```python
from build123d import *

# Parameters (mm, degrees)
F0_W     = 82.55
F0_H     = 57.15
F0_W_2   = 76.2
F0_H_2   = 50.8
F1_DEPTH = 152.4
F2_W     = 6.35
F2_H     = 57.15
F3_DEPTH = 50.8
F4_W     = 50.8
F4_H     = 6.35
F5_DEPTH = 50.8
F7_DEPTH = 118.618


with BuildPart() as f1:
    # F0 (on Front) → F1 (new body)
    with BuildSketch(Plane.XZ):
        with Locations((3.728271, -19.37303)):
            Rectangle(F0_W, F0_H)
        with Locations((3.728271, -19.37303)):
            Rectangle(F0_W_2, F0_H_2, mode=Mode.SUBTRACT)
    extrude(amount=F1_DEPTH)

    # F2 (on face) → F3 (join)
    with BuildSketch(Plane.YZ.offset(45.003271)):
        with Locations((-3.175, -19.37303)):
            Rectangle(F2_W, F2_H)
    extrude(amount=F3_DEPTH)

    # F4 (on face) → F5 (join)
    with BuildSketch(Plane.XZ.offset(6.35)):
        with Locations((70.403271, -44.77303)):
            Rectangle(F4_W, F4_H)
        with Locations((70.403271, 6.02697)):
            Rectangle(F4_W, F4_H)
    extrude(amount=F5_DEPTH)

    # F6 (on face) → F7 (cut)
    with BuildSketch(Plane.XY.offset(9.20197)):
        Polygon((95.803271, -6.35), (45.003271, -57.15), (95.803271, -57.15), align=None)
    extrude(amount=-F7_DEPTH, mode=Mode.SUBTRACT)


solid = f1.part
```
Input: part model. Units: mm. Frame: model coordinates. A direction names the side the tool comes from. Give positions to 0.01 mm unless a question says otherwise; leave off trailing zeros. Order: outer loops, then holes, each group sorted by start corner. A loop starts at its lowest first (then second) coordinate and runs counter-clockwise, first axis right, second up. Notation, with made-up numbers: M 61.5,67.25 L 112.5,67.25 A19 cw 112.5,71.25 Z; hole C 82.25,26.25 d4. An arc over 180 degrees is marked long. Return JSON: item names as keys, results as strings.
Item 1: Ray query, probe 1 along X at (y, z) = (-30.5, -10.5); probe 2 along Z at (x, y) = (-23.5, -36); probe 3 along X at (y, z) = (-21.5, 4.5). Return the intervals inside material, ascending.
Solutions:
{"probe 1": "-37.55 to -34.37, 41.83 to 45", "probe 2": "-47.95 to -44.77, 6.03 to 9.2", "probe 3": "-37.55 to -34.37, 41.83 to 80.65"}
Item 2: Cut plane D-D (x = 62). Return loops of the section in (y, z), then the cut area to 3 significant figures.
Solutions:
{"outline": "M -40.15,-47.95 L 0,-47.95 L 0,9.2 L -40.15,9.2 L -40.15,2.85 L -6.35,2.85 L -6.35,-41.6 L -40.15,-41.6 Z", "area": "792 mm^2"}
Item 3: Pull-direction query (X, two-part tool) for faces 1 (the flat face through (95.803, -3, -20)), 2 (the flat face through (-37.547, -75, -20)), 3 (the flat face through (3, -75, -44.773)), 4 (the flat face through (41.828, -75, -20)); classes: +X half, -X half, draft (parallel to the pull), parting line (faces both ways), or undercut.
Solutions:
{"face 1": "+X half", "face 2": "-X half", "face 3": "undercut", "face 4": "undercut"}
Item 4: Cut plane B-B (x = -1.5). Return loops of the section in (y, z).
Solutions:
{"outline": "M -152.4,-47.95 L 0,-47.95 L 0,-44.77 L -152.4,-44.77 Z; M -152.4,6.03 L 0,6.03 L 0,9.2 L -152.4,9.2 Z"}
Item 5: Cut plane C-C (y = -83). Return loops of the section in (x, z).
Solutions:
{"outline": "M -37.55,-47.95 L 45,-47.95 L 45,9.2 L -37.55,9.2 Z; hole M -34.37,-44.77 L 41.83,-44.77 L 41.83,6.03 L -34.37,6.03 Z"}
Item 6: Cut plane A-A (z = -11.5). Return loops of the section in (x, y).
Solutions:
{"outline": "M -37.55,-152.4 L -34.37,-152.4 L -34.37,0 L -37.55,0 Z; M 41.83,-152.4 L 45,-152.4 L 45,-6.35 L 95.8,-6.35 L 95.8,0 L 41.83,0 Z"}
Item 7: Access query for faces 5 (the flat face through (3, -75, 6.027)), 6 (the flat face through (13, -75, -47.948)), 7 (the flat face through (45.003, -78, -20)). Directions: +Z, -Z, +X, -X, +Y, -Y. A direction counts if a zero-diameter tool reaches every point of the face in a straight line with its end or side. Return the directions, or none.
Solutions:
{"face 5": "+Y, -Y", "face 6": "-Z, +X, -X, +Y, -Y", "face 7": "+X, -Y"}
Item 8: First-contact query: P1, Ø4, axis at x = 79.5, z = 0, coming from the -Y side; P2, Ø5, axis at y = -110.5, z = -8.5, coming from the +X side. Flat tips, straight axial feed; report the tip coordinate or a pass-through.
Solutions:
{"P1": "y = -6.35", "P2": "x = 45"}
